Verification items for the finished model (mm, model axes). Face numbers are marked on the shaded views. A direction names the side the tool comes from. Give positions to 0.01 mm unless a question says otherwise; leave off trailing zeros. Loops run counter-clockwise (first coordinate to the right, second up) from the corner with the lowest first, then second, coordinate; pieces in that order, holes last. Notation, with made-up numbers: (-39.75, -20) -> (-27.75, -20) arc R27 ccw to (-27.75, 16) -> close; hole circle Ø2 at (-21, 39.5). An arc over 180 degrees is marked (long way). Answer in a Markdown table with one row per item. Add a question column.
Q1. Section check A-A on x = -13.75. Enter the section's corners in (y, z).
Q2. Set-up check for the marked faces 1, 2 and 3: record each of +Z, -Z, +X, -X, +Y, -Y from which the full face is reachable in a straight line by a thin tool's end or side.
Q3. Material ranges on probe 1 along Y at (x, z) = (-13.75, 1.25); probe 2 along Y at (x, z) = (-13.75, 3.3); probe 3 along Y at (x, z) = (15.5, 5), recorded low to high.
Q4. Section check C-C on y = 20.15. Enter the section's corners in (x, z).
Q5. Gauge pin test, flat ends, axial feed: P1, Ø5, axis at x = -9, y = 10.5, coming from the -Z side; P2, Ø5, axis at x = -13.75, y = -19.7, coming from the -Z side; P3, Ø3, axis at x = -6.5, z = 2.5, coming from the -Y side; P4, Ø6.5, axis at x = 4, y = -74, coming from the -Z side. Record the tip position at first contact, or that the pin passes through.
Q6. Section check D-D on y = -6.1. Enter the section's corners in (x, z) (3 decimals), and give its area (3 significant figures).
Q7. Section check B-B on z = 1. Enter the section's corners in (x, y) (3 decimals).
```python
from build123d import *

# Parameters (mm, degrees)
SKETCH1_R           = 4.2
SKETCH1_R_2         = 9.6
BOSS_EXTRUDE1_DEPTH = 2
SKETCH2_W           = 40
SKETCH2_H           = 2
CUT_EXTRUDE1_DEPTH  = 1
SKETCH4_R           = 2
SKETCH4_R_2         = 9.6
BOSS_EXTRUDE3_DEPTH = 2
SKETCH5_W           = 40
SKETCH5_H           = 4
BOSS_EXTRUDE4_DEPTH = 2.3
SKETCH7_W           = 40
SKETCH7_H           = 57.5
SKETCH7_R           = 4
BOSS_EXTRUDE6_DEPTH = 4


with BuildPart() as part:
    # Sketch1 → Boss-Extrude1 (new body)
    with BuildSketch(Plane.XY):
        with BuildLine():
            Line((20, -29), (-20, -29))
            Line((-20, -29), (-20, 26))
            ThreePointArc((-20, 26), (-19.121320344, 28.121320344), (-17, 29))
            Line((-17, 29), (17, 29))
            ThreePointArc((17, 29), (19.121320344, 28.121320344), (20, 26))
            Line((20, 26), (20, -29))
        make_face()
        with Locations((-13.75, 20.15)):
            Circle(SKETCH1_R, mode=Mode.SUBTRACT)
        with Locations((13.75, 20.15)):
            Circle(SKETCH1_R, mode=Mode.SUBTRACT)
        with Locations((-13.75, -19.7)):
            Circle(SKETCH1_R, mode=Mode.SUBTRACT)
        with Locations((0, 8.8)):
            Circle(SKETCH1_R_2, mode=Mode.SUBTRACT)
        with Locations((-5.725, -6.1)):
            Circle(SKETCH1_R, mode=Mode.SUBTRACT)
        with Locations((5.725, -6.1)):
            Circle(SKETCH1_R, mode=Mode.SUBTRACT)
        with BuildLine():
            Line((11.314, -23.121389192), (7.240917629, -20.221389192))
            ThreePointArc((7.240917629, -20.221389192), (6.255528438, -14.364), (12.112917629, -13.378610808))
            Line((12.112917629, -13.378610808), (16.186, -16.278610808))
            ThreePointArc((16.186, -16.278610808), (17.171389192, -22.136), (11.314, -23.121389192))
        make_face(mode=Mode.SUBTRACT)
    extrude(amount=BOSS_EXTRUDE1_DEPTH)

    # Sketch2 → Cut-Extrude1 (cut)
    with BuildSketch(Plane.XZ.offset(29)):
        with Locations((0, 1)):
            Rectangle(SKETCH2_W, SKETCH2_H)
    extrude(amount=-CUT_EXTRUDE1_DEPTH, mode=Mode.SUBTRACT)

    # Sketch4 → Boss-Extrude3 (add)
    with BuildSketch(Plane.XY.offset(2)):
        with BuildLine():
            Line((-17, 29), (17, 29))
            ThreePointArc((17, 29), (19.121320344, 28.121320344), (20, 26))
            Line((20, 26), (20, -28))
            Line((20, -28), (-20, -28))
            Line((-20, -28), (-20, 26))
            ThreePointArc((-20, 26), (-19.121320344, 28.121320344), (-17, 29))
        make_face()
        with Locations((-13.75, -19.7)):
            Circle(SKETCH4_R, mode=Mode.SUBTRACT)
        with Locations((-13.75, 20.15)):
            Circle(SKETCH4_R, mode=Mode.SUBTRACT)
        with Locations((13.75, 20.15)):
            Circle(SKETCH4_R, mode=Mode.SUBTRACT)
        with Locations((13.75, -19.7)):
            Circle(SKETCH4_R, mode=Mode.SUBTRACT)
        with Locations((0, 8.8)):
            Circle(SKETCH4_R_2, mode=Mode.SUBTRACT)
    extrude(amount=BOSS_EXTRUDE3_DEPTH)

    # Sketch5 → Boss-Extrude4 (add)
    with BuildSketch(Plane.XY.offset(4)):
        with Locations((0, -26)):
            Rectangle(SKETCH5_W, SKETCH5_H)
    extrude(amount=BOSS_EXTRUDE4_DEPTH)

    # Sketch7 → Boss-Extrude6 (add)
    with BuildSketch(Plane.XY.offset(6.3)):
        with Locations((0, -52.75)):
            Rectangle(SKETCH7_W, SKETCH7_H)
        with Locations((4, -74)):
            Circle(SKETCH7_R, mode=Mode.SUBTRACT)
    extrude(amount=BOSS_EXTRUDE6_DEPTH)


solid = part.part
```
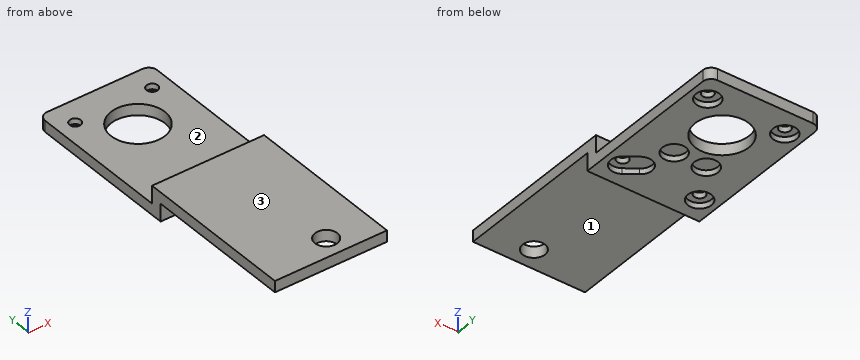
Taken from the geometry:
| question | item | result |
|---|---|---|
| 1 | outline | (-81.5, 6.3) -> (-28, 6.3) -> (-28, 0) -> (-23.9, 0) -> (-23.9, 2) -> (-21.7, 2) -> (-21.7, 4) -> (-24, 4) -> (-24, 10.3) -> (-81.5, 10.3) -> close; (-17.7, 2) -> (-15.5, 2) -> (-15.5, 0) -> (15.95, 0) -> (15.95, 2) -> (18.15, 2) -> (18.15, 4) -> (-17.7, 4) -> close; (22.15, 2) -> (24.35, 2) -> (24.35, 0) -> (29, 0) -> (29, 4) -> (22.15, 4) -> close |
| 2 | face 1 | -Z, +X, -X, -Y |
| 2 | face 2 | +Z, +X, -X, +Y |
| 2 | face 3 | +Z, +X, -X, +Y, -Y |
| 3 | probe 1 | y = -28 to -23.9, -15.5 to 15.95, 24.35 to 29 |
| 3 | probe 2 | y = -28 to -21.7, -17.7 to 18.15, 22.15 to 29 |
| 3 | probe 3 | y = -28 to -24 |
| 4 | outline | (-20, 0) -> (-17.95, 0) -> (-17.95, 2) -> (-15.75, 2) -> (-15.75, 4) -> (-20, 4) -> close; (-11.75, 2) -> (-9.55, 2) -> (-9.55, 0) -> (9.55, 0) -> (9.55, 2) -> (11.75, 2) -> (11.75, 4) -> (-11.75, 4) -> close; (15.75, 2) -> (17.95, 2) -> (17.95, 0) -> (20, 0) -> (20, 4) -> (15.75, 4) -> close |
| 5 | P1 | stops at z = 0 |
| 5 | P2 | stops at z = 2 |
| 5 | P3 | stops at y = -28 |
| 5 | P4 | passes through |
| 6 | outline | (-20, 0) -> (-9.925, 0) -> (-9.925, 2) -> (-1.525, 2) -> (-1.525, 0) -> (1.525, 0) -> (1.525, 2) -> (9.925, 2) -> (9.925, 0) -> (20, 0) -> (20, 4) -> (-20, 4) -> close |
| 6 | area | 126 mm² |
| 7 | outline | (-20, -28) -> (20, -28) -> (20, 26) arc R3 ccw to (17, 29) -> (-17, 29) arc R3 ccw to (-20, 26) -> close; hole circle Ø8.4 at (-13.75, -19.7); hole circle Ø8.4 at (-13.75, 20.15); hole circle Ø8.4 at (-5.725, -6.1); hole circle Ø19.2 at (0, 8.8); hole circle Ø8.4 at (5.725, -6.1); hole (7.241, -20.221) -> (11.314, -23.121) arc R4.2 ccw to (16.186, -16.279) -> (12.113, -13.379) arc R4.2 ccw to start; hole circle Ø8.4 at (13.75, 20.15) |
